Geometry check sheet. Reference: the model listing, model coordinates, mm. Give positions to 0.01 mm unless a question says otherwise; leave off trailing zeros. Write each loop counter-clockwise with the first axis right and the second up, starting at its lowest first coordinate (ties: lowest second). Pieces come first, ordered by that corner, then holes. Notation, with made-up numbers: M -27,23 L 12,23 A23 ccw 12,60 Z; hole C 78.5,74 d7. An arc over 180 degrees is marked long. One line per item, written item: value. Start each with the question number.
1. Release check for a two-part mould opening along Z. For faces 1 (the face through (1.5, 42.6, 35.1)), 2 (the face through (-2.25, -39, -80)), 3 (the face through (1.479, 48.59, -83.077)) record: pulls with the +Z half, pulls with the -Z half, needs draft (parallel to the pull), parting line crosses it, or undercut.
2. Cross-section at C-C on z = -3. Record the cut outline in (x, y).
3. Cross-section at D-D on x = 1.1. Count the separate pieces of the cut face and the enclosed holes in it, then the cut area to 3 significant figures.
4. Cross-section at B-B on z = -47. Record the cut outline in (x, y) (3 decimals), then the cut area to 3 significant figures.
5. Scan lines: line 1 (Y direction, x = 1.65, z = 27.5); line 2 (Z direction, x = 1.8, y = -5.5); line 3 (Y direction, x = 1.7, z = -86). Record each from-to range of solid material in increasing order.
6. Gauge pin test, flat ends, axial feed: pin 1 (1.5 mm diameter, centred on x = -1, z = -31.5, fed in from -Y); pin 2 (1.8 mm diameter, centred on x = -1, z = -77, fed in from +Y); pin 3 (1.8 mm diameter, centred on x = -1.5, y = -38.5, fed in from +Z); pin 4 (0.7 mm diameter, centred on x = -1.5, z = 77.5, fed in from -Y). Record the tip position at first contact, or that the pin passes through.
7. Cross-section at A-A on y = 29.5. Record the cut outline in (x, z).
from build123d import *

# Parameters (mm, degrees)
SKETCH_1_W           = 120
SKETCH_1_H           = 83
SKETCH_1_H_2         = 33
EXTRUDE_2_DEPTH      = 3
SKETCH_2_R           = 1.65
SKETCH_2_R_2         = 20
CUT_EXTRUDE_1_DEPTH  = 3
SKETCH_3_R           = 1.65
CUT_EXTRUDE_2_DEPTH  = 10
SKETCH_4_R           = 1.65
CUT_EXTRUDE_3_DEPTH  = 5
CUT_EXTRUDE_6_DEPTH  = 3
SKETCH_9_W           = 5
SKETCH_9_H           = 5
EXTRUDE_4_DEPTH      = 2.25
SKETCH_8_R           = 1.65
CUT_EXTRUDE_9_DEPTH  = 7
SKETCH_11_R          = 9
CUT_EXTRUDE_10_DEPTH = 10


with BuildPart() as part:
    # 草图1 → 凸台-拉伸2 (new body)
    with BuildSketch(Plane(origin=(0, 0, 0), x_dir=(0, 0, -1), z_dir=(1, 0, 0))):
        with Locations((0, -16.5)):
            Rectangle(SKETCH_1_W, SKETCH_1_H)
        with Locations((0, 41.5)):
            Rectangle(SKETCH_1_W, SKETCH_1_H_2)
        with BuildLine():
            Line((-60, -58), (-60, 58))
            ThreePointArc((-60, 58), (-83.334523779, 48.334523779), (-93, 25))
            Line((-93, 25), (-93, -25))
            ThreePointArc((-93, -25), (-83.334523779, -48.334523779), (-60, -58))
        make_face()
        with BuildLine():
            ThreePointArc((60, 58), (83.334523779, 48.334523779), (93, 25))
            Line((93, 25), (93, -25))
            ThreePointArc((93, -25), (83.334523779, -48.334523779), (60, -58))
            Line((60, -58), (60, 58))
        make_face()
    extrude(amount=EXTRUDE_2_DEPTH)

    # 草图2 → 切除-拉伸1 (cut)
    with BuildSketch(Plane(origin=(3, 0, 0), x_dir=(0, 0, -1), z_dir=(1, 0, 0))):
        with Locations((-52.5, -39.650635095)):
            Circle(SKETCH_2_R)
        with Locations((40, -18)):
            Circle(SKETCH_2_R_2)
        with Locations((-40, -18)):
            Circle(SKETCH_2_R_2)
        with Locations((-52.5, 3.650635095)):
            Circle(SKETCH_2_R)
        with Locations((-65, -18)):
            Circle(SKETCH_2_R)
        with Locations((-27.5, -39.650635095)):
            Circle(SKETCH_2_R)
        with Locations((-15, -18)):
            Circle(SKETCH_2_R)
        with Locations((15, -18)):
            Circle(SKETCH_2_R)
        with Locations((27.5, 3.650635095)):
            Circle(SKETCH_2_R)
        with Locations((52.5, 3.650635095)):
            Circle(SKETCH_2_R)
        with Locations((65, -18)):
            Circle(SKETCH_2_R)
        with Locations((52.5, -39.650635095)):
            Circle(SKETCH_2_R)
        with Locations((27.5, -39.650635095)):
            Circle(SKETCH_2_R)
        with Locations((-27.5, 3.650635095)):
            Circle(SKETCH_2_R)
        with Locations((-40, 22)):
            Circle(SKETCH_2_R)
        with Locations((40, 22)):
            Circle(SKETCH_2_R)
    extrude(amount=-CUT_EXTRUDE_1_DEPTH, mode=Mode.SUBTRACT)

    # 草图3 → 切除-拉伸2 (cut)
    with BuildSketch(Plane(origin=(3, 0, 0), x_dir=(0, 0, -1), z_dir=(1, 0, 0))):
        with Locations((-10, -51)):
            Circle(SKETCH_3_R)
        with Locations((10, -51)):
            Circle(SKETCH_3_R)
    extrude(amount=-CUT_EXTRUDE_2_DEPTH, mode=Mode.SUBTRACT)

    # 草图4 → 切除-拉伸3 (cut)
    with BuildSketch(Plane.ZY):
        with Locations((86, 15)):
            Circle(SKETCH_4_R)
        with Locations((86, -15)):
            Circle(SKETCH_4_R)
        with Locations((-86, 15)):
            Circle(SKETCH_4_R)
        with Locations((-86, -15)):
            Circle(SKETCH_4_R)
    extrude(amount=-CUT_EXTRUDE_3_DEPTH, mode=Mode.SUBTRACT)

    # 草图6 → 切除-拉伸6 (cut)
    with BuildSketch(Plane.ZY):
        Polygon((-25, 32.5), (-33, 32.5), (-53, 52.5), (-45, 52.5), align=None)
        Polygon((0, 49.270509831), (-8.816778784, 42.864745084), (-5.44906896, 32.5), (5.44906896, 32.5), (8.816778784, 42.864745084), align=None)
        Polygon((-10, 32.5), (-18, 32.5), (-38, 52.5), (-30, 52.5), align=None)
        Polygon((38, 52.5), (30, 52.5), (10, 32.5), (18, 32.5), align=None)
        Polygon((53, 52.5), (45, 52.5), (25, 32.5), (33, 32.5), align=None)
    extrude(amount=-CUT_EXTRUDE_6_DEPTH, mode=Mode.SUBTRACT)

    # 草图9 → 凸台-拉伸4 (add)
    with BuildSketch(Plane.ZY):
        with Locations((-78, -39.5)):
            Rectangle(SKETCH_9_W, SKETCH_9_H)
        with Locations((78, -39.5)):
            Rectangle(SKETCH_9_W, SKETCH_9_H)
    extrude(amount=EXTRUDE_4_DEPTH)

    # 草图8 → 切除-拉伸9 (cut)
    with BuildSketch(Plane(origin=(3, 0, 0), x_dir=(0, 0, -1), z_dir=(1, 0, 0))):
        with Locations((78, -39.5)):
            Circle(SKETCH_8_R)
        with Locations((-78, -39.5)):
            Circle(SKETCH_8_R)
    extrude(amount=-CUT_EXTRUDE_9_DEPTH, mode=Mode.SUBTRACT)

    # 草图11 → 切除-拉伸10 (cut)
    with BuildSketch(Plane(origin=(3, 0, 0), x_dir=(0, 0, -1), z_dir=(1, 0, 0))):
        with Locations((-65, 33)):
            Circle(SKETCH_11_R)
        with Locations((65, 33)):
            Circle(SKETCH_11_R)
    extrude(amount=-CUT_EXTRUDE_10_DEPTH, mode=Mode.SUBTRACT)


solid = part.part
Report:
1. face 1: undercut
1. face 2: needs draft
1. face 3: pulls with the -Z half
2. outline: M 0,-58 L 3,-58 L 3,32.5 L 0,32.5 Z; M 0,47.09 L 3,47.09 L 3,58 L 0,58 Z
3. separate pieces: 1
3. enclosed holes: 31
3. area: 16,600 mm^2
4. outline: M 0,-58 L 3,-58 L 3,-36.735 L 0,-36.735 Z; M 0,0.735 L 3,0.735 L 3,46.5 L 0,46.5 Z; M 0,52.5 L 3,52.5 L 3,58 L 0,58 Z
4. area: 218 mm^2
5. line 1: y = -58 to -41.3, -38 to -33.61, -2.39 to 2, 5.3 to 32.5, 35 to 42, 50 to 58
5. line 2: z = -93 to -55.61, -24.39 to 24.39, 55.61 to 93
5. line 3: y = -45.32 to -16.65, -13.35 to 13.35, 16.65 to 45.32
6. pin 1: passes through
6. pin 2: stops at y = -37
6. pin 3: stops at z = 80.5
6. pin 4: stops at y = -42
7. outline: M 0,-92.69 L 3,-92.69 L 3,-73.29 L 0,-73.29 Z; M 0,-56.71 L 3,-56.71 L 3,56.71 L 0,56.71 Z; M 0,73.29 L 3,73.29 L 3,92.69 L 0,92.69 Z
